Autodesk Inventor part; units mm, degrees
ref_plane "YZ Plane" through (0, 0, 0) normal (1, 0, 0) x (0, 1, 0)
ref_plane "XZ Plane" through (0, 0, 0) normal (0, 1, 0) x (-1, 0, 0)
ref_plane "XY Plane" through (0, 0, 0) normal (0, 0, 1) x (1, 0, 0)
sketch "스케치2" plane through (0, 0, 0) normal (0, 1, 0) x (-1, 0, 0)
  line L0 (65, -2.8774) -> (0, -2.8774)
  line L1 (0, -2.8774) -> (0, -117.8774)
  line L2 (0, -117.8774) -> (65, -117.8774)
  line L3 (65, -117.8774) -> (65, -2.8774)
  line L4 (61, -6.8774) -> (4, -6.8774)
  line L5 (4, -6.8774) -> (4, -113.8774)
  line L6 (4, -113.8774) -> (61, -113.8774)
  line L7 (61, -113.8774) -> (61, -6.8774)
  point P0 (0, 0)
  dimension "d0" = 65
  dimension "d1" = 115
  dimension "d2" = 4
extrude "돌출1" add sketch "스케치2" along normal blind 30
extrude "돌출2" add sketch "스케치2" along normal blind 5 contours L7 L6 L5 L4
properties part number "gps_case_2"
Design review of the part built by this model. Coordinates are the model's own, in mm. A direction names the side the tool comes from. Coordinates: 2 decimals unless noted, no trailing zeros. Loops run counter-clockwise (first coordinate to the right, second up) from the corner with the lowest first, then second, coordinate; pieces in that order, holes last.
Q1. We need section B-B on z = -77. State the section outline as (x, y) points, and give its area (3 significant figures).
Reported:
outline: (-65, 0) - (0, 0) - (0, 30) - (-4, 30) - (-4, 5) - (-61, 5) - (-61, 30) - (-65, 30) - close
area: 525 mm2
Q2. Tool access review of faces 4 (the face through (-61, 17, -61)), 5 (the face through (-3, 30, -56)): name each direction out of +Z, -Z, +X, -X, +Y, -Y from which nothing blocks a thin tool from reaching the whole face with its end or side.
Reported:
face 4: +Y
face 5: +Z, -Z, +X, -X, +Y
Q3. We need section C-C on x = -19. State the section outline as (y, z) points, and give its area (3 significant figures).
Reported:
outline: (0, -117.88) - (30, -117.88) - (30, -113.88) - (5, -113.88) - (5, -6.88) - (30, -6.88) - (30, -2.88) - (0, -2.88) - close
area: 775 mm2
Q4. We need section A-A on y = 25.25. State the section outline as (x, z) points.
Reported:
outline: (-65, -117.88) - (0, -117.88) - (0, -2.88) - (-65, -2.88) - close; hole (-61, -113.88) - (-4, -113.88) - (-4, -6.88) - (-61, -6.88) - close
Q5. For pin 1 (6 mm diameter, centred on x = -31, z = -42, fed in from -Y); pin 2 (2 mm diameter, centred on x = -22, z = -101, fed in from +Y), all flat-tipped, find the tip position at first contact; note any pin that passes through.
Reported:
pin 1: stops at y = 0
pin 2: stops at y = 5
Q6. The part is to be moulded in two halves that separate along X. For faces 1 (the face through (-4, 17, -60)), 2 (the face through (-65, 15, -61)), 3 (the face through (-32, 15, -117.877)), say which applies: +X half, -X half, draft (parallel to the pull), parting line (faces both ways), or undercut.
Reported:
face 1: undercut
face 2: -X half
face 3: draft
Q7. To check wall thickness, follow line 1 (Z direction, x = -11.5, y = 28); line 2 (X direction, y = 24, z = -55); line 3 (Y direction, x = -42, z = -79). State the ranges of each line that lie inside material, in increasing order.
Reported:
line 1: z = -117.88 to -113.88, -6.88 to -2.88
line 2: x = -65 to -61, -4 to 0
line 3: y = 0 to 5
